from build123d import *

# Parameters (mm, degrees)
F0_W      = 10
F0_H      = 10
F1_DEPTH  = 10
F2_R      = 4
F3_DEPTH  = 5
F4_R      = 4
F5_DEPTH  = 5
F6_R      = 4
F7_DEPTH  = 5
F8_R      = 4
F9_DEPTH  = 5
F10_R     = 4
F11_DEPTH = 5
F12_R     = 4
F13_DEPTH = 5


with BuildPart() as f1:
    # F0 (on Top) → F1 (new body)
    with BuildSketch(Plane.XY):
        Rectangle(F0_W, F0_H)
    extrude(amount=F1_DEPTH)

    # F2 (on face) → F3 (join)
    with BuildSketch(Plane.YZ.offset(5)):
        with Locations((0, 5)):
            Circle(F2_R)
    extrude(amount=F3_DEPTH)

    # F4 (on face) → F5 (join)
    with BuildSketch(Plane(origin=(0, 0, 0), x_dir=(1, 0, 0), z_dir=(0, 0, -1))):
        Circle(F4_R)
    extrude(amount=F5_DEPTH)

    # F6 (on face) → F7 (join)
    with BuildSketch(Plane(origin=(-5, 0, 0), x_dir=(0, -1, 0), z_dir=(-1, 0, 0))):
        with Locations((0, 5)):
            Circle(F6_R)
    extrude(amount=F7_DEPTH)

    # F8 (on face) → F9 (join)
    with BuildSketch(Plane.XY.offset(10)):
        Circle(F8_R)
    extrude(amount=F9_DEPTH)

    # F10 (on face) → F11 (join)
    with BuildSketch(Plane(origin=(0, 5, 0), x_dir=(-1, 0, 0), z_dir=(0, 1, 0))):
        with Locations((0, 5)):
            Circle(F10_R)
    extrude(amount=F11_DEPTH)

    # F12 (on face) → F13 (join)
    with BuildSketch(Plane.XZ.offset(5)):
        with Locations((0, 5)):
            Circle(F12_R)
    extrude(amount=F13_DEPTH)


solid = f1.part
Work out the finished part from the listing and answer in its coordinate system (mm). A direction names the side the tool comes from. Round coordinates to 2 decimals unless told otherwise and drop trailing zeros. Write each loop counter-clockwise with the first axis right and the second up, starting at its lowest first coordinate (ties: lowest second). Pieces come first, ordered by that corner, then holes.
1) A cutting plane is placed at C-C (z = -3). Give the vertices of the cut face in (x, y), plus the area to 3 significant figures.
2) A cutting plane is placed at D-D (y = 6). Give the vertices of the cut face in (x, z).
3) Given pin 1 Ø1 at (x, z) = (-3.5, -2) entering from +Y; pin 2 Ø1.5 at (x, z) = (-5, 9.5) entering from -Y; pin 3 Ø5 at (x, z) = (7, 1.5) entering from +Y; pin 4 Ø12 at (x, z) = (2, 1) entering from +Y, each flat-ended and moving along its own axis, determine where each tip first touches the part or whether it passes through.
4) A cutting plane is placed at A-A (x = 0). Give the vertices of the cut face in (y, z), plus the area to 3 significant figures.
5) Straight lines are drawn through the part: line 1 (Z direction, x = -4, y = 1.25); line 2 (X direction, y = -4.5, z = 1); line 3 (Y direction, x = -2.5, z = -1.75). For each, find the intervals that lie inside material, in ascending order.
6) A tool of negligible diameter and unlimited length cuts with its end or side. For faces 1 (the flat face through (5, -0.1, 0.5)), 2 (the flat face through (-0.1, -5, 0.5)), 3 (the flat face through (-0.1, 5, 0.5)), from which of +Z, -Z, +X, -X, +Y, -Y can it reach the whole face along a straight path? Write none if from no direction.
Completed:
1. outline: circle Ø8 at (0, 0)
1. area: 50.3 mm2
2. outline: circle Ø8 at (0, 5)
3. pin 1: stops at y = 2.65
3. pin 2: stops at y = -5
3. pin 3: stops at y = 5
3. pin 4: stops at y = 10
4. outline: (-10, 1) - (-5, 1) - (-5, 0) - (-4, 0) - (-4, -5) - (4, -5) - (4, 0) - (5, 0) - (5, 1) - (10, 1) - (10, 9) - (5, 9) - (5, 10) - (4, 10) - (4, 15) - (-4, 15) - (-4, 10) - (-5, 10) - (-5, 9) - (-10, 9) - close
4. area: 260 mm2
5. line 1: z = 0 to 10
5. line 2: x = -5 to 5
5. line 3: y = -3.12 to 3.12
6. face 1: +X
6. face 2: -Y
6. face 3: +Y
